Part model, mm, in its own coordinate system. Face numbers are marked on the shaded views. Round coordinates to 2 decimals unless told otherwise and drop trailing zeros. Loops run counter-clockwise (first coordinate to the right, second up) from the corner with the lowest first, then second, coordinate; pieces in that order, holes last. Notation, with made-up numbers: M 56,44.5 L 103,44.5 A23 cw 103,62.5 Z; hole C -18.75,66.5 d7. An arc over 180 degrees is marked long. Answer as CSV lines item,"result". Start each with the question number.
Item 1: Band-saw the part on A-A (y = 155). Give the cut face in (x, z).
Item 2: Wall check: line 1 (Z direction, x = 3.5, y = -198). Give the ranges that are in metal, low to high.
Item 3: Drop flat-ended pins along their axis: pin 1 Ø8 at (x, z) = (-23.5, 53.5) entering from +Y; pin 2 Ø8 at (x, z) = (-11, 38) entering from +Y. Give the stop position or say it passes through.
Item 4: Mould opens along X. For the marked faces 1, 2 and 3 say: pulls with the +X half, pulls with the -X half, needs draft (parallel to the pull), parting line crosses it, or undercut.
Item 5: Band-saw the part on C-C (z = 24). Give the cut face in (x, y).
Item 6: Band-saw the part on B-B (x = -15). Give the cut face in (y, z).
Item 7: Band-saw the part on D-D (x = 13.5). Give the cut face in (y, z), and give its area (3 significant figures).
```python
from build123d import *

# Parameters (mm, degrees)
F0_W     = 80
F0_H     = 600
F0_R     = 5
F1_DEPTH = 40
F2_DEPTH = 70


with BuildPart() as f1:
    # F0 (on Top) → F1 (new body)
    with BuildSketch(Plane.XY):
        Rectangle(F0_W, F0_H)
        with Locations((-15, 105)):
            Circle(F0_R, mode=Mode.SUBTRACT)
        with Locations((-15, 155)):
            Circle(F0_R, mode=Mode.SUBTRACT)
        with Locations((-15, 155)):
            Circle(F0_R)
        with Locations((-15, 105)):
            Circle(F0_R)
    extrude(amount=-F1_DEPTH)

    # F0 (on Top) → F2 (join)
    with BuildSketch(Plane.XY):
        with Locations((-15, 155)):
            Circle(F0_R)
        with Locations((-15, 105)):
            Circle(F0_R)
    extrude(amount=F2_DEPTH)


solid = f1.part
```
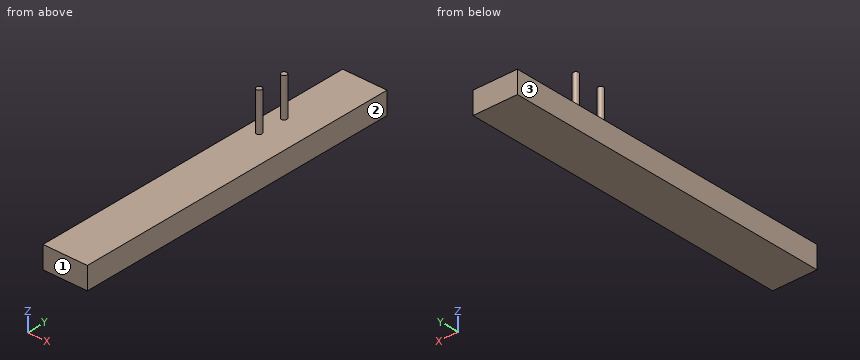
Answer block:
1,outline,"M -40,-40 L 40,-40 L 40,0 L -10,0 L -10,70 L -20,70 L -20,0 L -40,0 Z"
2,line 1,"z = -40 to 0"
3,pin 1,"stops at y = 157.18"
3,pin 2,"stops at y = 160"
4,face 1,"needs draft"
4,face 2,"pulls with the +X half"
4,face 3,"pulls with the -X half"
5,outline,"C -15,105 d10; C -15,155 d10"
6,outline,"M -300,-40 L 300,-40 L 300,0 L 160,0 L 160,70 L 150,70 L 150,0 L 110,0 L 110,70 L 100,70 L 100,0 L -300,0 Z"
7,outline,"M -300,-40 L 300,-40 L 300,0 L -300,0 Z"
7,area,"24,000 mm^2"
